Autodesk Inventor part; units mm, degrees
ref_plane "YZ Plane" through (0, 0, 0) normal (1, 0, 0) x (0, 1, 0)
ref_plane "XZ Plane" through (0, 0, 0) normal (0, 1, 0) x (-1, 0, 0)
ref_plane "XY Plane" through (0, 0, 0) normal (0, 0, 1) x (1, 0, 0)
sketch "草图1" plane through (0, 0, 0) normal (0, 0, 1) x (1, 0, 0)
  circle A0 centre (0, 0) radius 4.25
  dimension "d0" = 8.5
extrude "拉伸1" add sketch "草图1" along normal blind 25
sketch "草图2" plane through (0, 0, 0) normal (0, 0, -1) x (-1, 0, 0)
  line L0 (-25, 25) -> (25, 25)
  line L1 (25, 25) -> (25, -25)
  line L2 (25, -25) -> (-25, -25)
  line L3 (-25, -25) -> (-25, 25)
  circle A0 centre (0, 0) radius 4.25
  line L4 (-25, 25) -> (25, -25) construction
  line L5 (25, 25) -> (-25, -25) construction
  dimension "d3" = 50
  dimension "d4" = 50
extrude "拉伸2" add sketch "草图2" along normal blind 10 contours L0 L1 L2 L3 | A0
sketch "草图3" plane through (0, 0, 0) normal (0, 0, 1) x (1, 0, 0)
  circle A0 centre (0, 0) radius 15
  dimension "d7" = 30
extrude "拉伸3" cut sketch "草图3" against normal blind 2
sketch "草图4" plane through (0, 0, -2) normal (0, 0, 1) x (1, 0, 0)
  circle A0 centre (0, 0) radius 10
  dimension "d10" = 20
extrude "拉伸4" cut sketch "草图4" against normal blind 1
sketch "草图5" plane through (0, 0, -3) normal (0, 0, 1) x (1, 0, 0)
  circle A0 centre (0, 0) radius 7.5
  dimension "d13" = 15
extrude "拉伸5" add sketch "草图5" along normal blind 2
sketch "草图6" plane through (0, 0, -1) normal (0, 0, 1) x (1, 0, 0)
  circle A0 centre (0, 0) radius 4.25
extrude "拉伸6" add sketch "草图6" along normal blind 2
sketch "草图7" plane through (0, 0, -10) normal (0, 0, -1) x (-1, 0, 0)
  line L0 (-20, 20) -> (20, 20)
  line L1 (20, 20) -> (20, -20)
  line L2 (20, -20) -> (-20, -20)
  line L3 (-20, -20) -> (-20, 20)
  line L4 (-20, 20) -> (20, -20) construction
  line L5 (20, 20) -> (-20, -20) construction
  point P0 (0, 0)
  dimension "d18" = 40
  dimension "d19" = 40
extrude "拉伸7" add sketch "草图7" along normal blind 25
sketch "草图8" plane through (0, 0, -35) normal (0, 0, -1) x (-1, 0, 0)
  line L0 (25, -25) -> (25, 25)
  line L1 (-25, 25) -> (25, 25)
  line L2 (25, 25) -> (25, -25)
  line L3 (25, -25) -> (-25, -25)
  line L4 (-25, -25) -> (-25, 25)
  circle A0 centre (0, 0) radius 7.5
  line L5 (-25, 25) -> (25, -25) construction
  line L6 (25, 25) -> (-25, -25) construction
  dimension "d22" = 50
  dimension "d23" = 50
extrude "拉伸8" add sketch "草图8" along normal blind 10 contours L3 L4 L1 L0 | A0
chamfer "倒角1" distance 5 angle 45 12 edges at (20, -20, -22.5) (25, -25, -5) (25, -25, -40) (-25, -25, -40) (-20, -20, -22.5) (-25, -25, -5) (25, 25, -5) (20, 20, -22.5) (25, 25, -40) (-20, 20, -22.5) (-25, 25, -5) (-25, 25, -40)
properties part number "步进电机2"
Could you check a few things on this model? Use its own coordinates, in mm. A direction names the side the tool comes from. Give positions to 0.01 mm unless a question says otherwise; leave off trailing zeros. Order: outer loops, then holes, each group sorted by start corner. A loop starts at its lowest first (then second) coordinate and runs counter-clockwise, first axis right, second up.
Item 1: I'm going to push flat-ended pins straight in: pin 1 (7.5 mm diameter, centred on x = 4.5, z = -28.5, fed in from -Y); pin 2 (8 mm diameter, centred on x = 11.5, y = -9, fed in from +Z); pin 3 (20 mm diameter, centred on y = -5, z = -22.5, fed in from -X). Where does each tip first touch, or does it pass through?
Item 2: If we section it at D-D, the plane y = 16.5: Write out the boundary of the cut face in (x, z).
Item 3: If we mould it in two halves opening along Y, with no side actions, what happens to faces 6 (the face through (-11, -11, 0)), 7 (the face through (-14.985, 0.66, -0.986)), 8 (the face through (23, 22, -5)), 9 (the face through (-18, -17, -23))? For each: pulls with the +Y half, pulls with the -Y half, needs draft (parallel to the pull), parting line crosses it, or undercut.
Item 4: If we section it at A-A, the plane y = 0: Write out the boundary of the cut face in (x, z).
Item 5: I need wall thicknesses on line 1 (Y direction, x = 0, z = -2.4); line 2 (Z direction, x = -18.5, y = 19.5); line 3 (Z direction, x = 15.5, y = -5). Which ranges of each line are inside material? Lowest first, please.
Item 6: If we section it at C-C, the plane z = -23: Write out the boundary of the cut face in (x, y), plus the area to 3 significant figures.
Item 7: For faces 1 (the face through (-17, 18, -23)), 2 (the face through (0, -22, -10)), 3 (the face through (0, -20, -22)), 4 (the face through (2.285, -3.584, 11.818)), 5 (the face through (18, -17, -22)), which set-ups out of +Z, -Z, +X, -X, +Y, -Y let a thin tool reach every point of the face, with its end or its side?
Values:
1. pin 1: stops at y = -20
1. pin 2: stops at z = 0
1. pin 3: stops at x = -20
2. outline: (-25, -45) - (25, -45) - (25, -35) - (18.5, -35) - (18.5, -10) - (25, -10) - (25, 0) - (-25, 0) - (-25, -10) - (-18.5, -10) - (-18.5, -35) - (-25, -35) - close
3. face 6: needs draft
3. face 7: undercut
3. face 8: pulls with the +Y half
3. face 9: pulls with the -Y half
4. outline: (-25, -45) - (25, -45) - (25, -35) - (20, -35) - (20, -10) - (25, -10) - (25, 0) - (15, 0) - (15, -2) - (10, -2) - (10, -3) - (7.5, -3) - (7.5, -1) - (4.25, -1) - (4.25, 25) - (-4.25, 25) - (-4.25, -1) - (-7.5, -1) - (-7.5, -3) - (-10, -3) - (-10, -2) - (-15, -2) - (-15, 0) - (-25, 0) - (-25, -10) - (-20, -10) - (-20, -35) - (-25, -35) - close
5. line 1: y = -25 to -10, -7.5 to 7.5, 10 to 25
5. line 2: z = -45 to -35, -10 to 0
5. line 3: z = -45 to 0
6. outline: (-20, -15) - (-15, -20) - (15, -20) - (20, -15) - (20, 15) - (15, 20) - (-15, 20) - (-20, 15) - close
6. area: 1,550 mm2
7. face 1: -X, +Y
7. face 2: none
7. face 3: +X, -X, -Y
7. face 4: +Z
7. face 5: +X, -Y
